Job drawing, mm, ordinate dimensions from the low corner. One solid piece. A direction names the side the tool comes from. Round coordinates to 2 decimals unless told otherwise and drop trailing zeros. Write each loop counter-clockwise with the first axis right and the second up, starting at its lowest first coordinate (ties: lowest second). Pieces come first, ordered by that corner, then holes.
1) Saw through at C-C (y = 61). Write the cut outline in (x, z).
2) Which spindle directions (+Z, -Z, +X, -X, +Y, -Y) get a long thin tool onto all of the face, cutting with end or side? Do the marked faces 4 and 5. Say none if no direction does.
3) Flat gauge pins, fed straight in: pin 1 (4 mm diameter, centred on x = 46.5, y = 49, fed in from -Z); pin 2 (3 mm diameter, centred on x = 26.5, y = 65.5, fed in from +Z). Where does each tip first touch, or does it go through?
4) Pull direction Y, two halves, no side cores. Call the marked faces 1, 2 and 3: +Y half, -Y half, draft (parallel to the pull), parting line (faces both ways), or undercut.
5) Saw through at B-B (x = 8). Write the cut outline in (y, z), plus the area to 3 significant figures.
6) Saw through at A-A (z = 88). Write the cut outline in (x, y), plus the area to 3 significant figures.
7) Wall check: probe 1 along Y at (x, z) = (10, 81); probe 2 along Z at (x, y) = (23.5, 107). Give the ranges that are in metal, low to high.
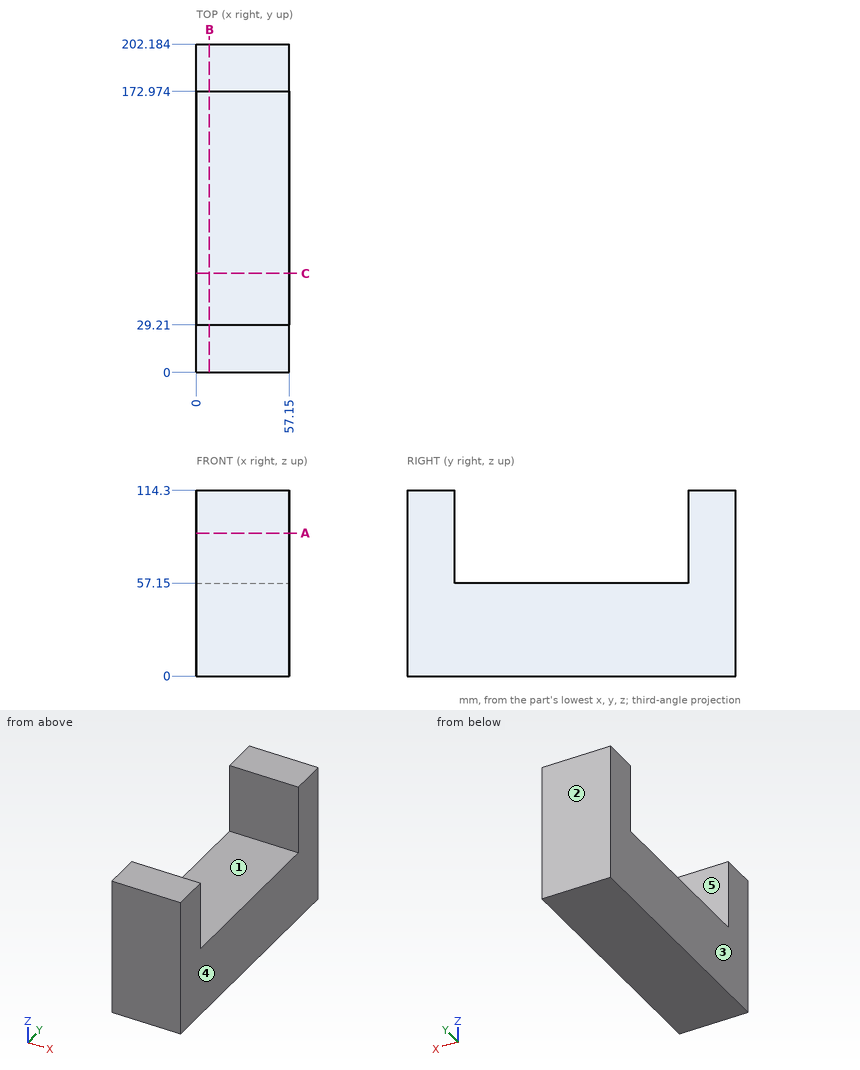
Evaluation:
1. outline: (0, 0) - (57.15, 0) - (57.15, 57.15) - (0, 57.15) - close
2. face 4: +Z, -Z, +X, +Y, -Y
2. face 5: +Z, +X, -X
3. pin 1: stops at z = 0
3. pin 2: stops at z = 57.15
4. face 1: undercut
4. face 2: +Y half
4. face 3: draft
5. outline: (0, 0) - (202.18, 0) - (202.18, 114.3) - (172.97, 114.3) - (172.97, 57.15) - (29.21, 57.15) - (29.21, 114.3) - (0, 114.3) - close
5. area: 14,900 mm2
6. outline: (0, 0) - (57.15, 0) - (57.15, 29.21) - (0, 29.21) - close; (0, 172.97) - (57.15, 172.97) - (57.15, 202.18) - (0, 202.18) - close
6. area: 3,340 mm2
7. probe 1: y = 0 to 29.21, 172.97 to 202.18
7. probe 2: z = 0 to 57.15
